Can you work these out from the model? Positions are in its coordinate system, mm. Give positions to 0.01 mm unless a question says otherwise; leave off trailing zeros. Write each loop counter-clockwise with the first axis right and the second up, starting at its lowest first coordinate (ties: lowest second). Pieces come first, ordered by that corner, then holes.
1. Suppose I cut it at B-B (z = -37.25). Please give me the cut outline in (x, y), and give its area (3 significant figures).
2. Suppose I cut it at A-A (y = -1.1). Please give me the cut outline in (x, z).
3. Suppose I cut it at C-C (z = -31). Please give me the cut outline in (x, y), and give its area (3 significant figures).
4. If I drill on probe 1 along X at (y, z) = (-1.6, -35.5); probe 2 along X at (y, z) = (-0.8, -36.25), over which ranges is the centre line in solid material (lowest first)?
```python
from build123d import *

# Parameters (mm, degrees)
F0_W        = 114.3
F0_H        = 9.525
F1_DEPTH    = 2.0066
F2_R        = 5.08
F3_T1_DEPTH = 27.2073812379
F4_R        = 5.08
F5_T1_DEPTH = 27.2073812379


# Not quite as in the source:
# - a fillet or chamfer that OpenCascade refuses, or shapes differently, is made with other operations: its cross-section is extruded or revolved along the edge and cut away or added


with BuildPart() as f1:
    # F0 (on Front) → F1 (new body)
    with BuildSketch(Plane.XZ):
        with Locations((-10.4238372296, -33.6832711485)):
            Rectangle(F0_W, F0_H)
    extrude(amount=F1_DEPTH)

    # F2
    f2_edges = [f1.edges().sort_by_distance(p)[0] for p in [
        (46.726163, -1.0033, -28.920771),
    ]]
    fillet(f2_edges, radius=F2_R)

    # F3: fillet of radius 5.08 on 1 edges, made by hand

    # F3_s2 → F3_t1 (cut)
    with BuildSketch(Plane.XZ.offset(-12.6003906189)):
        with BuildLine():
            ThreePointArc((46.7261627704, -34.0007711485), (45.0461106879, -37.1757711485), (41.6860065228, -38.4457711485))
            Line((41.6860065228, -38.4457711485), (46.7261627704, -38.4457711485))
            Line((46.7261627704, -38.4457711485), (46.7261627704, -34.0007711485))
        make_face()
    extrude(amount=F3_T1_DEPTH, mode=Mode.SUBTRACT)

    # F4
    f4_edges = [f1.edges().sort_by_distance(p)[0] for p in [
        (-67.573837, -1.0033, -28.920771),
    ]]
    fillet(f4_edges, radius=F4_R)

    # F5: fillet of radius 5.08 on 1 edges, made by hand

    # F5_s2 → F5_t1 (cut)
    with BuildSketch(Plane.XZ.offset(-12.6003906189)):
        with BuildLine():
            ThreePointArc((-67.5738372296, -34.0007711485), (-65.8937851471, -37.1757711485), (-62.533680982, -38.4457711485))
            Line((-62.533680982, -38.4457711485), (-67.5738372296, -38.4457711485))
            Line((-67.5738372296, -38.4457711485), (-67.5738372296, -34.0007711485))
        make_face()
    extrude(amount=F5_T1_DEPTH, mode=Mode.SUBTRACT)


solid = f1.part
```
Checks:
1. outline: (-65.81, -2.01) - (44.96, -2.01) - (44.96, 0) - (-65.81, 0) - close
1. area: 222 mm2
2. outline: (-67.57, -34) arc R5.08 ccw to (-62.53, -38.45) - (41.69, -38.45) arc R5.08 ccw to (46.73, -34) arc R5.08 ccw to (41.65, -28.92) - (-62.49, -28.92) arc R5.08 ccw to start
3. outline: (-66.59, -2.01) - (45.75, -2.01) - (45.75, 0) - (-66.59, 0) - close
3. area: 225 mm2
4. probe 1: x = -67.14 to 46.3
4. probe 2: x = -66.72 to 45.87
